from build123d import *

# Parameters (mm, degrees)
SKETCH087_W         = 108
SKETCH087_H         = 108
PAD038_DEPTH        = 78
POCKET039_DEPTH     = 78.001
FILLET006_R         = 8
POCKET043_DEPTH     = 78.001
REVOLUTION017_ANGLE = -180
REVOLUTION018_ANGLE = -180
REVOLUTION019_ANGLE = -180
SKETCH119_W         = 13.26
SKETCH119_H         = 8.92
POCKET059_DEPTH     = 2
SKETCH156_R         = 8.75
POCKET060_DEPTH     = 2
SKETCH157_R         = 8.75
POCKET061_DEPTH     = 2


with BuildPart() as part:
    # Sketch087 → Pad038 (new body)
    with BuildSketch(Plane.XY):
        with Locations((54, 54)):
            Rectangle(SKETCH087_W, SKETCH087_H)
    extrude(amount=PAD038_DEPTH)

    # Sketch107 (on Face6 of Pad038) → Pocket039 (cut, through all)
    with BuildSketch(Plane.XY.offset(78)):
        Polygon((2, 98), (10, 98), (10, 106), (98, 106), (98, 98), (106, 98), (106, 10), (98, 10), (98, 2), (10, 2), (10, 10), (2, 10), align=None)
    extrude(amount=-POCKET039_DEPTH, mode=Mode.SUBTRACT)

    # Fillet006
    fillet006_edges = [part.edges().sort_by_distance(p)[0] for p in [
        (0, 108, 39),
        (108, 108, 39),
        (108, 0, 39),
        (0, 0, 39),
    ]]
    fillet(fillet006_edges, radius=FILLET006_R)

    # Sketch115 (on Face5 of Fillet006) → Pocket043 (cut, through all)
    with BuildSketch(Plane.XY.offset(78)):
        Polygon((2, 100), (8, 100), (8, 106), align=None)
        Polygon((100, 106), (100, 100), (106, 100), align=None)
        Polygon((100, 2), (100, 8), (106, 8), align=None)
        Polygon((2, 8), (8, 8), (8, 2), align=None)
    extrude(amount=-POCKET043_DEPTH, mode=Mode.SUBTRACT)

    # Sketch116 → Revolution017 (revolve)
    with BuildSketch(Plane.XZ):
        with BuildLine():
            add(Edge.make_bspline(
                [(36, 57), (39, 57), (39, 64.5), (39, 72), (36, 72)],
                knots=[0, 0, 0, 1.570796, 1.570796, 3.141593, 3.141593, 3.141593], degree=2, weights=[1, 0.707107, 1, 0.707107, 1]))
            Line((36, 72), (36, 57))
        make_face()
    revolve(axis=Axis((36, 0, 57), (0, 0, 1)), revolution_arc=REVOLUTION017_ANGLE)

    # Sketch117 → Revolution018 (revolve)
    with BuildSketch(Plane.XZ):
        with BuildLine():
            add(Edge.make_bspline(
                [(72, 57), (75, 57), (75, 64.5), (75, 72), (72, 72)],
                knots=[0, 0, 0, 1.570796, 1.570796, 3.141593, 3.141593, 3.141593], degree=2, weights=[1, 0.707107, 1, 0.707107, 1]))
            Line((72, 72), (72, 57))
        make_face()
    revolve(axis=Axis((72, 0, 57), (0, 0, 1)), revolution_arc=REVOLUTION018_ANGLE)

    # Sketch118 → Revolution019 (revolve)
    with BuildSketch(Plane.XZ):
        with BuildLine():
            add(Edge.make_bspline(
                [(59, 52.5), (59, 55), (54, 55), (49, 55), (49, 52.5)],
                knots=[0, 0, 0, 1.570796, 1.570796, 3.141593, 3.141593, 3.141593], degree=2, weights=[1, 0.707107, 1, 0.707107, 1]))
            Line((49, 52.5), (59, 52.5))
        make_face()
    revolve(axis=Axis((59, 0, 52.5), (-1, 0, 0)), revolution_arc=REVOLUTION019_ANGLE)

    # Sketch119 → Pocket059 (cut)
    with BuildSketch(Plane(origin=(0, 108, 0), x_dir=(-1, 0, 0), z_dir=(0, 1, 0))):
        with Locations((-54, 34.46)):
            Rectangle(SKETCH119_W, SKETCH119_H)
    extrude(amount=-POCKET059_DEPTH, mode=Mode.SUBTRACT)

    # Sketch156 (on Face6 of Pocket059) → Pocket060 (cut)
    with BuildSketch(Plane.YZ.offset(108)):
        with Locations((54, 48)):
            Circle(SKETCH156_R)
    extrude(amount=-POCKET060_DEPTH, mode=Mode.SUBTRACT)

    # Sketch157 (on Face5 of Pocket060) → Pocket061 (cut)
    with BuildSketch(Plane(origin=(0, 0, 0), x_dir=(0, -1, 0), z_dir=(-1, 0, 0))):
        with Locations((-54, 48)):
            Circle(SKETCH157_R)
    extrude(amount=-POCKET061_DEPTH, mode=Mode.SUBTRACT)


with BuildPart() as part_1:
    # Body015 placement: moved
    add(part.part.moved(Location((0, 0, 106))))


solid = part_1.part
Work out the finished part from the listing and answer in its coordinate system (mm). A direction names the side the tool comes from. Give positions to 0.01 mm unless a question says otherwise; leave off trailing zeros. Loops run counter-clockwise (first coordinate to the right, second up) from the corner with the lowest first, then second, coordinate; pieces in that order, holes last. Notation, with made-up numbers: (88.25, 48) - (104.25, 48) arc R19 cw to (104.25, 68) - close; hole circle Ø3 at (14.5, 34). An arc over 180 degrees is marked (long way). Answer in a Markdown table with one row per item. Add a question column.
Q1. A tool of negligible diameter and unlimited length cuts with its end or side. For faces 1 (the flat face through (98, 6, 146)), 2 (the cylindrical face through (2.281, 105.594, 145.546)), from which of +Z, -Z, +X, -X, +Y, -Y can it reach the whole face along a straight path? Write none if from no direction.
Q2. The part is cut by section A-A (y = 95.5). Determine the outline of the cut face in (x, z), and give its area (3 significant figures).
Q3. Determine the mould class of faces 3 (the flat face through (53.4, 108, 135.8)), 4 (the cylindrical face through (105.594, 2.281, 145.546)), 5 (the flat face through (103, 8, 146)) for opening direction X: released by +X, released by -X, zero draft, split by the parting line, or undercut.
Q4. Consider line 1 along X through (y, z) = (51.5, 113); line 2 along Z through (x, y) = (106.75, 54). Determine where each line is inside the solid, lowest interval first.
Q5. The part is cut by section D-D (y = 54). Determine the outline of the cut face in (x, z).
Q6. Each of these flat-tipped pins is pushed along its axis until it touches: P1, Ø6.5, axis at x = 4, z = 163.5, coming from the -Y side; P2, Ø1.8, axis at x = 104, z = 134, coming from the -Y side; P3, Ø3, axis at x = 49, z = 142, coming from the +Y side. Where does it stop, or does it pass through?
Q7. The part is cut by section C-C (z = 122). State how many separate pieces and enclosed holes the cut face has, and give its area (3 significant figures).
Solution:
| question | item | result |
|---|---|---|
| 1 | face 1 | +Z, -Z |
| 1 | face 2 | +Z, -Z, -X, +Y |
| 2 | outline | (0, 106) - (2, 106) - (2, 184) - (0, 184) - close; (106, 106) - (108, 106) - (108, 184) - (106, 184) - close |
| 2 | area | 312 mm² |
| 3 | face 3 | zero draft |
| 3 | face 4 | released by +X |
| 3 | face 5 | undercut |
| 4 | line 1 | x = 0 to 2, 106 to 108 |
| 4 | line 2 | z = 106 to 145.25, 162.75 to 184 |
| 5 | outline | (0, 106) - (2, 106) - (2, 145.25) - (0, 145.25) - close; (0, 162.75) - (2, 162.75) - (2, 184) - (0, 184) - close; (106, 106) - (108, 106) - (108, 145.25) - (106, 145.25) - close; (106, 162.75) - (108, 162.75) - (108, 184) - (106, 184) - close |
| 6 | P1 | stops at y = 0.04 |
| 6 | P2 | stops at y = 0.63 |
| 6 | P3 | stops at y = 2 |
| 7 | separate pieces | 1 |
| 7 | enclosed holes | 5 |
| 7 | area | 977 mm² |
